Geometry check sheet. Reference: the model listing, model coordinates, mm. Face numbers are marked on the shaded views. A direction names the side the tool comes from. Coordinates: 2 decimals unless noted, no trailing zeros. Order: outer loops, then holes, each group sorted by start corner. A loop starts at its lowest first (then second) coordinate and runs counter-clockwise, first axis right, second up. Notation, with made-up numbers: (-36.75, 63.5) - (-10.75, 63.5) arc R31 cw to (-10.75, 100.5) - close; hole circle Ø4 at (77.25, -7.5). An arc over 180 degrees is marked (long way). Return JSON: item names as keys, results as strings. Group by question number.
Item 1: Section check B-B on x = -7.5. Enter the section's corners in (y, z) (3 decimals), then the cut area to 3 significant figures.
Item 2: Section check A-A on z = 16. Enter the section's corners in (x, y).
Item 3: Section check D-D on x = -5. Enter the section's corners in (y, z) (3 decimals).
Item 4: Section check C-C on y = -5.25. Enter the section's corners in (x, z), then the cut area to 3 significant figures.
Item 5: Gauge pin test, flat ends, axial feed: pin 1 (2 mm diameter, centred on y = -20.5, z = 11, fed in from -X); pin 2 (3 mm diameter, centred on x = -9.5, y = -3.5, fed in from +Z); pin 3 (9 mm diameter, centred on x = -16.5, z = 14.5, fed in from +Y). Record the tip position at first contact, or that the pin passes through.
Item 6: Tool access check on the marked faces 1 and 2. Record the directions out of +Z, -Z, +X, -X, +Y, -Y that give a thin tool (end or side, any length) a straight path to the whole face; none if there is none.
Item 7: Scan lines: probe 1 along Z at (x, y) = (-19.61, -24.55); probe 2 along Y at (x, z) = (-10.75, 5.5); probe 3 along Z at (x, y) = (-1.75, -3.5). Record each from-to range of solid material in increasing order.
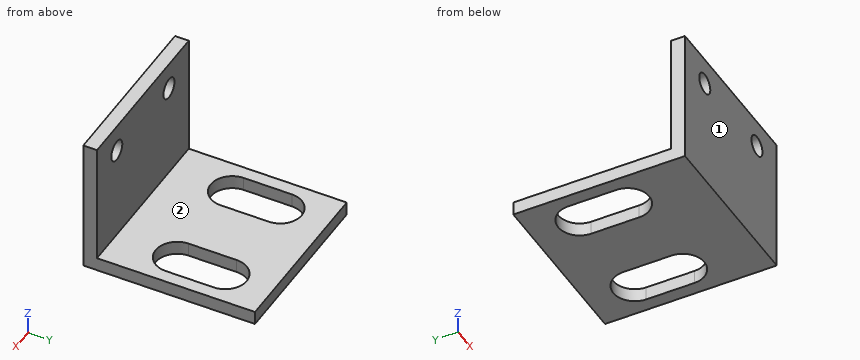
from build123d import *

# Parameters (mm, degrees)
F1_DEPTH = 25
F3_DEPTH = 25
F4_R     = 1.5
F5_DEPTH = 25


with BuildPart() as f1:
    # F0 (on Right) → F1 (new body)
    with BuildSketch(Plane.YZ):
        Polygon((-25, 0), (0, 0), (0, 2), (-23, 2), (-23, 20), (-25, 20), align=None)
    extrude(amount=-F1_DEPTH)

    # F2 (on face) → F3 (cut)
    with BuildSketch(Plane.XY.offset(2)):
        with BuildLine():
            Line((-16.875, -14), (-16.875, -7))
            ThreePointArc((-16.875, -7), (-20, -3.875), (-23.125, -7))
            Line((-23.125, -7), (-23.125, -14))
            ThreePointArc((-23.125, -14), (-20, -17.125), (-16.875, -14))
        make_face()
        with BuildLine():
            Line((-1.875, -14), (-1.875, -7))
            ThreePointArc((-1.875, -7), (-5, -3.875), (-8.125, -7))
            Line((-8.125, -7), (-8.125, -14))
            ThreePointArc((-8.125, -14), (-5, -17.125), (-1.875, -14))
        make_face()
    extrude(amount=-F3_DEPTH, mode=Mode.SUBTRACT)

    # F4 (on face) → F5 (cut)
    with BuildSketch(Plane(origin=(0, -23, 0), x_dir=(-1, 0, 0), z_dir=(0, 1, 0))):
        with Locations((5.39, 16)):
            Circle(F4_R)
        with Locations((19.61, 16)):
            Circle(F4_R)
    extrude(amount=-F5_DEPTH, mode=Mode.SUBTRACT)


solid = f1.part
Computed:
{
 "1": {"outline": "(-25, 0) - (-15.875, 0) - (-15.875, 2) - (-23, 2) - (-23, 20) - (-25, 20) - close; (-5.125, 0) - (0, 0) - (0, 2) - (-5.125, 2) - close", "area": "64.5 mm²"},
 "2": {"outline": "(-25, -25) - (-21.11, -25) - (-21.11, -23) - (-25, -23) - close; (-18.11, -25) - (-6.89, -25) - (-6.89, -23) - (-18.11, -23) - close; (-3.89, -25) - (0, -25) - (0, -23) - (-3.89, -23) - close"},
 "3": {"outline": "(-25, 0) - (-17.125, 0) - (-17.125, 2) - (-23, 2) - (-23, 14.552) - (-25, 14.552) - close; (-25, 17.448) - (-23, 17.448) - (-23, 20) - (-25, 20) - close; (-3.875, 0) - (0, 0) - (0, 2) - (-3.875, 2) - close"},
 "4": {"outline": "(-25, 0) - (-22.59, 0) - (-22.59, 2) - (-25, 2) - close; (-17.41, 0) - (-7.59, 0) - (-7.59, 2) - (-17.41, 2) - close; (-2.41, 0) - (0, 0) - (0, 2) - (-2.41, 2) - close", "area": "29.3 mm²"},
 "5": {"pin 1": "passes through", "pin 2": "stops at z = 2", "pin 3": "stops at y = -23"},
 "6": {"face 1": "+Z, -Z, +X, -X, -Y", "face 2": "+Z, +X, -X, +Y"},
 "7": {"probe 1": "z = 0 to 14.5, 17.5 to 20", "probe 2": "y = -25 to -23", "probe 3": "z = 0 to 2"}
}
